```python
from build123d import *

# Parameters (mm, degrees)
SKETCH_1_R           = 1.5
EXTRUDE_1_DEPTH      = 8
EXTRUDE_2_DEPTH      = 19
EXTRUDE_2_DEPTH_BACK = 11
FILLET_1_R           = 2
FILLET_2_R           = 2
FILLET_4_R           = 2
FILLET_5_R           = 2
SKETCH_3_W           = 10
SKETCH_3_H           = 10
SKETCH_3_R           = 3
CUT_EXTRUDE_1_DEPTH  = 8
SKETCH_3_2_W         = 10
SKETCH_3_2_H         = 10
SKETCH_3_2_R         = 3
EXTRUDE_3_DEPTH      = 7
SKETCH_3_3_W         = 10
SKETCH_3_3_H         = 10
SKETCH_3_3_R         = 3
CUT_EXTRUDE_2_DEPTH  = 1


with BuildPart() as part:
    # Sketch 1 → Extrude 1 (new body)
    with BuildSketch(Plane.XY):
        with BuildLine():
            Line((-15, 0), (15, 0))
            Line((15, 0), (15, 15.404082058))
            ThreePointArc((15, 15.404082058), (4.5, 35), (15, 54.595917942))
            Line((15, 54.595917942), (15, 60))
            Line((15, 60), (8, 60))
            Line((8, 60), (-15, 15))
            Line((-15, 15), (-15, 0))
        make_face()
        with Locations((-10, 5)):
            Circle(SKETCH_1_R, mode=Mode.SUBTRACT)
        with Locations((10, 5)):
            Circle(SKETCH_1_R, mode=Mode.SUBTRACT)
    extrude(amount=EXTRUDE_1_DEPTH)

    # Sketch 2 → Extrude 2 (add, two sides: drawn at the far end of the back side and taken through both)
    with BuildSketch(Plane.XY.offset(-EXTRUDE_2_DEPTH_BACK)):
        with BuildLine():
            Line((-12.166399205, 20.544001556), (8, 60))
            Line((8, 60), (15, 60))
            Line((15, 60), (15, 54.595917942))
            ThreePointArc((15, 54.595917942), (4.805132127, 38.777552052), (9.462778171, 20.544001556))
            Line((9.462778171, 20.544001556), (-12.166399205, 20.544001556))
        make_face()
    extrude(amount=EXTRUDE_2_DEPTH + EXTRUDE_2_DEPTH_BACK)

    # Fillet 1
    fillet_1_edges = [part.edges().sort_by_distance(p)[0] for p in [
        (-1.351810517, 20.544001556, 19),
    ]]
    fillet(fillet_1_edges, radius=FILLET_1_R)

    # Fillet 2
    fillet_2_edges = [part.edges().sort_by_distance(p)[0] for p in [
        (-1.351810517, 20.544001556, -11),
    ]]
    fillet(fillet_2_edges, radius=FILLET_2_R)

    # Fillet 4
    fillet_4_edges = [part.edges().sort_by_distance(p)[0] for p in [
        (8, 60, 4),
    ]]
    fillet(fillet_4_edges, radius=FILLET_4_R)

    # Fillet 5
    fillet_5_edges = [part.edges().sort_by_distance(p)[0] for p in [
        (15, 0, 4),
        (-15, 0, 4),
    ]]
    fillet(fillet_5_edges, radius=FILLET_5_R)

    # Sketch 3 → Cut-Extrude 1 (cut)
    # profile 1 of 2: a face of its own
    with BuildSketch(Plane(origin=(0, 0, 0), x_dir=(-1, 0, 0), z_dir=(0, 0, -1))):
        with Locations((-10, 5)):
            Rectangle(SKETCH_3_W, SKETCH_3_H)
        with Locations((-10, 5)):
            Circle(SKETCH_3_R, mode=Mode.SUBTRACT)
    # profile 2 of 2: a face of its own
    with BuildSketch(Plane(origin=(0, 0, 0), x_dir=(-1, 0, 0), z_dir=(0, 0, -1))):
        with Locations((10, 5)):
            Rectangle(SKETCH_3_W, SKETCH_3_H)
        with Locations((10, 5)):
            Circle(SKETCH_3_R, mode=Mode.SUBTRACT)
    extrude(amount=-CUT_EXTRUDE_1_DEPTH, mode=Mode.SUBTRACT)


with BuildPart() as cut_extrude_1_piece_1:
    # of the separate pieces the step leaves, piece 1, a body of its own (cut_extrude_1_pieces)
    add(part.part.solids().sort_by_distance((-12.166399205, 20.544001556, 0))[0])



with BuildPart() as cut_extrude_1_piece_2:
    # of the separate pieces the step leaves, piece 2, a body of its own (cut_extrude_1_pieces)
    add(part.part.solids().sort_by_distance((-13, 5, 0))[0])


with BuildPart() as cut_extrude_1_piece_3:
    # of the separate pieces the step leaves, piece 3, a body of its own (cut_extrude_1_pieces)
    add(part.part.solids().sort_by_distance((7, 5, 0))[0])


with BuildPart() as cut_extrude_1_piece_1_1:
    add(cut_extrude_1_piece_1.part)

    add(cut_extrude_1_piece_2.part)  # Extrude 3 merges Cut-Extrude 1 piece 2

    add(cut_extrude_1_piece_3.part)  # Extrude 3 merges Cut-Extrude 1 piece 3
    # Sketch 3_2 → Extrude 3 (add)
    # profile 1 of 2: a face of its own
    with BuildSketch(Plane(origin=(0, 0, 0), x_dir=(-1, 0, 0), z_dir=(0, 0, -1))):
        with Locations((-10, 5)):
            Rectangle(SKETCH_3_2_W, SKETCH_3_2_H)
        with Locations((-10, 5)):
            Circle(SKETCH_3_2_R, mode=Mode.SUBTRACT)
    # profile 2 of 2: a face of its own
    with BuildSketch(Plane(origin=(0, 0, 0), x_dir=(-1, 0, 0), z_dir=(0, 0, -1))):
        with Locations((10, 5)):
            Rectangle(SKETCH_3_2_W, SKETCH_3_2_H)
        with Locations((10, 5)):
            Circle(SKETCH_3_2_R, mode=Mode.SUBTRACT)
    extrude(amount=-EXTRUDE_3_DEPTH)

    # Sketch 3_3 → Cut-Extrude 2 (cut)
    # profile 1 of 2: a face of its own
    with BuildSketch(Plane(origin=(0, 0, 0), x_dir=(-1, 0, 0), z_dir=(0, 0, -1))):
        with Locations((-10, 5)):
            Rectangle(SKETCH_3_3_W, SKETCH_3_3_H)
        with Locations((-10, 5)):
            Circle(SKETCH_3_3_R, mode=Mode.SUBTRACT)
    # profile 2 of 2: a face of its own
    with BuildSketch(Plane(origin=(0, 0, 0), x_dir=(-1, 0, 0), z_dir=(0, 0, -1))):
        with Locations((10, 5)):
            Rectangle(SKETCH_3_3_W, SKETCH_3_3_H)
        with Locations((10, 5)):
            Circle(SKETCH_3_3_R, mode=Mode.SUBTRACT)
    extrude(amount=-CUT_EXTRUDE_2_DEPTH, mode=Mode.SUBTRACT)


solid = cut_extrude_1_piece_1_1.part
```
The listing builds one solid part. Answer for the finished solid, in the listing's coordinates (mm). A direction names the side the tool comes from. Round coordinates to 2 decimals unless told otherwise and drop trailing zeros. Loops run counter-clockwise (first coordinate to the right, second up) from the corner with the lowest first, then second, coordinate; pieces in that order, holes last.
Q1. Given pin 1 Ø1.8 at (x, y) = (11, 6.5) entering from -Z; pin 2 Ø3 at (x, y) = (8.5, 5.5) entering from +Z; pin 3 Ø5 at (y, z) = (26, 5) entering from -X, each flat-ended and moving along its own axis, determine where each tip first touches the part or whether it passes through.
Q2. Section C-C, the plane x = -10 is taken. Determine the outline of the cut face in (y, z).
Q3. For a pull along Y with two mould halves and no side action, classify faces 4 (the face through (2, 37, -11)), 5 (the face through (-7.7, 7.3, 7)), 6 (the face through (-1.503, 21.145, -10.43)) as released by +Y, released by -Y, zero draft, split by the parting line, or undercut.
Q4. Which of the six approach directions +Z, -Z, +X, -X, +Y, -Y give full straight-line access (tool end or side, diameter ignored) to faces 1 (the face through (11.3, 3.7, 8)), 2 (the face through (-1, 20.544, -5)), 3 (the face through (12.3, 7.3, 7))?
Q5. Section D-D, the plane x = 10.5 is taken. Determine the outline of the cut face in (y, z).
Q6. Find the intervals of material crossed by line 1 (Y direction, x = 10, z = 2); line 2 (Z direction, x = 6, y = 4.5); line 3 (Y direction, x = -10, z = 4), in increasing order.
Q7. Section B-B, the plane z = 4.5 is taken. Determine the outline of the cut face in (x, y).
Q8. Section A-A, the plane x = -3.5 is taken. Determine the outline of the cut face in (y, z), then the cut area to 3 significant figures.
Completed:
1. pin 1: stops at z = 0
1. pin 2: stops at z = 8
1. pin 3: stops at x = -10.66
2. outline: (0, 1) - (2, 1) - (2, 0) - (3.5, 0) - (3.5, 8) - (2, 8) - (2, 7) - (0, 7) - close; (6.5, 0) - (8, 0) - (8, 1) - (10, 1) - (10, 0) - (20.54, 0) - (20.54, -9) arc R2 ccw to (22.54, -11) - (24.78, -11) - (24.78, 19) - (22.54, 19) arc R2 ccw to (20.54, 17) - (20.54, 8) - (10, 8) - (10, 7) - (8, 7) - (8, 8) - (6.5, 8) - close
3. face 4: zero draft
3. face 5: undercut
3. face 6: released by -Y
4. face 1: +Z, +X, -X, -Y
4. face 2: -Z, +X, -X, -Y
4. face 3: +Z
5. outline: (0, 1) - (2.04, 1) - (2.04, 0) - (3.59, 0) - (3.59, 8) - (2.04, 8) - (2.04, 7) - (0, 7) - close; (6.41, 0) - (7.96, 0) - (7.96, 1) - (10, 1) - (10, 0) - (19.3, 0) - (19.3, 8) - (10, 8) - (10, 7) - (7.96, 7) - (7.96, 8) - (6.41, 8) - close; (50.7, -11) - (60, -11) - (60, 19) - (50.7, 19) - close
6. line 1: y = 0 to 3.5, 6.5 to 19.88, 50.12 to 60
6. line 2: z = 1 to 7
6. line 3: y = 0 to 3.5, 6.5 to 24.78
7. outline: (-15, 0) - (15, 0) - (15, 15.4) arc R23.54 cw to (15, 54.6) - (15, 60) - (9.22, 60) arc R2 ccw to (7.44, 58.91) - (-15, 15) - close; hole circle Ø3 at (-10, 5); hole circle Ø3 at (10, 5)
8. outline: (0, 0) - (20.54, 0) - (20.54, -9) arc R2 ccw to (22.54, -11) - (37.5, -11) - (37.5, 19) - (22.54, 19) arc R2 ccw to (20.54, 17) - (20.54, 8) - (0, 8) - close
8. area: 671 mm2
